```python
from build123d import *

# Parameters (mm, degrees)
SKETCH2_R              = 1.65
CUT_EXTRUDE_3_6_DEPTH  = 4.5
CHAMFER_1_SIZE         = 1
SKETCH3_R              = 1
CUT_EXTRUDE_3_20_DEPTH = 25


with BuildPart() as part:
    # Sketch1 → Revolve 696 (revolve)
    with BuildSketch(Plane(origin=(0, 0, 0), x_dir=(0, 0, -1), z_dir=(1, 0, 0)), mode=Mode.PRIVATE) as revolve_696_sk:
        Polygon((-7.5, 12.7), (25, 12.7), (25, 17.6), (18, 17.6), (18, 18.6), (-10, 18.6), (-10, 3.65), (-7.5, 3.65), align=None)
    revolve(revolve_696_sk.sketch.rotate(Axis((0, 0, 0), (0, 0, -1)), 90), axis=Axis((0, 0, 0), (0, 0, -1)))

    # Sketch2 → Крепление к двигателю (винт с потайной головкой М3х6) (cut)
    with BuildSketch(Plane.XY.offset(10)):
        with Locations((8.5, 0)):
            Circle(SKETCH2_R)
        with Locations((-8.5, 0)):
            Circle(SKETCH2_R)
    extrude(amount=-CUT_EXTRUDE_3_6_DEPTH, mode=Mode.SUBTRACT)

    # Фаска 1
    chamfer_1_edges = [part.edges().sort_by_distance(p)[0] for p in [
        (6.85, 0, 10),
        (-10.15, 0, 10),
    ]]
    chamfer(chamfer_1_edges, length=CHAMFER_1_SIZE)

    # Sketch3 → Отверстие под саморез М3х20 (cut)
    with BuildSketch(Plane(origin=(0, 0, -25), x_dir=(-1, 0, 0), z_dir=(0, 0, -1))):
        with Locations((-10.606601718, 10.606601718)):
            Circle(SKETCH3_R)
        with Locations((10.606601718, 10.606601718)):
            Circle(SKETCH3_R)
        with Locations((10.606601718, -10.606601718)):
            Circle(SKETCH3_R)
        with Locations((-10.606601718, -10.606601718)):
            Circle(SKETCH3_R)
    extrude(amount=-CUT_EXTRUDE_3_20_DEPTH, mode=Mode.SUBTRACT)

    # Эскиз2 → Cut-Revolve 1559 (revolve, cut)
    with BuildSketch(Plane(origin=(0, 0, 0), x_dir=(0, 0, -1), z_dir=(1, 0, 0)), mode=Mode.PRIVATE) as cut_revolve_1559_sk:
        Polygon((-10, 18.6), (-10, 16.6), (13, 18.6), align=None)
    revolve(cut_revolve_1559_sk.sketch.rotate(Axis((0, 0, 10), (0, 0, -1)), 90), axis=Axis((0, 0, 10), (0, 0, -1)), mode=Mode.SUBTRACT)


solid = part.part
```
CAD build for the part. Positions are in the model's coordinates, mm. A direction names the side the tool comes from. Round coordinates to 2 decimals unless told otherwise and drop trailing zeros. Order: outer loops, then holes, each group sorted by start corner. A loop starts at its lowest first (then second) coordinate and runs counter-clockwise, first axis right, second up. Notation, with made-up numbers: (14, 21.25) - (64, 21.25) arc R37 cw to (64, 59.25) - close; hole circle Ø8 at (-19.75, 73.5). An arc over 180 degrees is marked (long way). Answer in a Markdown table with one row per item. Add a question column.
(1) Band-saw the part on A-A on y = 0. Count the separate pieces of the cut face and the enclosed holes in it, and give its area (3 significant figures).
(2) Band-saw the part on C-C on z = -17. List the corners of the cut face in (x, y), and give its area (3 significant figures).
(3) 3-axis set-ups, long thin cutter, end or side, ignore diameter. For faces 4 (the face through (-4, 0, 10)), 5 (the face through (-11, -11, 0)): which of +Z, -Z, +X, -X, +Y, -Y reach the whole face in a straight line?
(4) Mould opens along Y. For faces 1 (the face through (11, 14, -18)), 2 (the face through (-3, 3, 7.5)), 3 (the face through (9.999, -15.684, -15.465)) say: +Y half, -Y half, draft (parallel to the pull), parting line (faces both ways), or undercut.
(5) Band-saw the part on D-D on z = -2. List the corners of the cut face in (x, y), and give its area (3 significant figures).
(6) Band-saw the part on B-B on x = 0. List the corners of the cut face in (y, z).
(7) Probe L1, parallel to X at y = 11.5, z = -3; L2, parallel to Y at x = -9.5, z = 2; L3, parallel to X at y = -9, z = -22. List the from-to ranges inside material, lowest first. Write a range as [from, to].
(8) Drop flat-ended pins along their axis: pin 1 Ø1.5 at (x, z) = (-2.5, 5.5) entering from +Y; pin 2 Ø2 at (x, y) = (8.5, 0) entering from +Z; pin 3 Ø2 at (x, y) = (-10.5, 10.5) entering from -Z; pin 4 Ø1 at (y, z) = (13, -20.5) entering from -X. Give the stop position or say it passes through.
Data:
| question | item | result |
|---|---|---|
| 1 | separate pieces | 4 |
| 1 | enclosed holes | 0 |
| 1 | area | 380 mm^2 |
| 2 | outline | circle Ø37.2 at (0, 0); hole circle Ø25.4 at (0, 0); hole circle Ø2 at (-10.61, -10.61); hole circle Ø2 at (-10.61, 10.61); hole circle Ø2 at (10.61, -10.61); hole circle Ø2 at (10.61, 10.61) |
| 2 | area | 568 mm^2 |
| 3 | face 4 | +Z, +X, -X, +Y, -Y |
| 3 | face 5 | -Z |
| 4 | face 1 | draft |
| 4 | face 2 | undercut |
| 4 | face 3 | parting line |
| 5 | outline | circle Ø35.29 at (0, 0); hole circle Ø25.4 at (0, 0); hole circle Ø2 at (-10.61, -10.61); hole circle Ø2 at (-10.61, 10.61); hole circle Ø2 at (10.61, -10.61); hole circle Ø2 at (10.61, 10.61) |
| 5 | area | 459 mm^2 |
| 6 | outline | (-18.6, -18) - (-17.6, -18) - (-17.6, -25) - (-12.7, -25) - (-12.7, 7.5) - (-3.65, 7.5) - (-3.65, 10) - (-16.6, 10) - (-18.6, -13) - close; (3.65, 7.5) - (12.7, 7.5) - (12.7, -25) - (17.6, -25) - (17.6, -18) - (18.6, -18) - (18.6, -13) - (16.6, 10) - (3.65, 10) - close |
| 7 | L1 | x = [-13.5, -11.06], [-10.16, -5.39], [5.39, 10.16], [11.06, 13.5] |
| 7 | L2 | y = [-14.45, -8.43], [8.43, 14.45] |
| 7 | L3 | x = [-15.12, -8.96], [8.96, 15.12] |
| 8 | pin 1 | stops at y = 16.92 |
| 8 | pin 2 | passes through |
| 8 | pin 3 | stops at z = -25 |
| 8 | pin 4 | stops at x = -12.39 |
